```python
from build123d import *

# Parameters (mm, degrees)
SZKIC2_R                   = 3.3
SZKIC2_R_2                 = 8
WYTNIJ_WYCI_GNI_CIE1_DEPTH = 56.569775958


with BuildPart() as part:
    # Szkic1 → Obrót1 (revolve)
    with BuildSketch(Plane(origin=(0, 0, 0), x_dir=(0, 0, -1), z_dir=(1, 0, 0)), mode=Mode.PRIVATE) as obr_t1_sk:
        Polygon((0, 0), (44, 0), (44, 14), (10, 14), (10, 24), (0, 24), align=None)
    revolve(obr_t1_sk.sketch.rotate(Axis((0, 0, 0), (0, 0, -1)), 90), axis=Axis((0, 0, 0), (0, 0, -1)))

    # Szkic2 → Wytnij-wyciągnięcie1 (cut, through all)
    with BuildSketch(Plane.XY):
        with Locations((-13.435028843, 13.435028843)):
            Circle(SZKIC2_R)
        with Locations((0, 19)):
            Circle(SZKIC2_R)
        with Locations((13.435028843, 13.435028843)):
            Circle(SZKIC2_R)
        Circle(SZKIC2_R_2)
        with BuildLine():
            Line((-20, 13.266499161), (-20, -13.266499161))
            ThreePointArc((-20, -13.266499161), (-24, 0), (-20, 13.266499161))
        make_face()
        with BuildLine():
            Line((20, -13.266499161), (20, 13.266499161))
            ThreePointArc((20, 13.266499161), (24, 0), (20, -13.266499161))
        make_face()
    wytnij_wyci_gni_cie1 = extrude(amount=-WYTNIJ_WYCI_GNI_CIE1_DEPTH, mode=Mode.SUBTRACT)

    # Lustro1: Wytnij-wyciągnięcie1 across plane
    add(wytnij_wyci_gni_cie1.mirror(Plane.ZX), mode=Mode.SUBTRACT)


solid = part.part
```
The model under review builds one solid part; all positions refer to its coordinate system, in mm. A direction names the side the tool comes from. Coordinates: 2 decimals unless noted, no trailing zeros. Write each loop counter-clockwise with the first axis right and the second up, starting at its lowest first coordinate (ties: lowest second). Pieces come first, ordered by that corner, then holes. Notation, with made-up numbers: (-28.75, -4.5) - (22.25, -4.5) arc R18 ccw to (22.25, 5.5) - close; hole circle Ø7 at (-20.75, -16.75). An arc over 180 degrees is marked (long way). Answer in a Markdown table with one row per item. Add a question column.
Q1. Draft analysis for pull direction Y (two halves, no side actions). For faces 1 (the face through (9, 0, 0)), 2 (the face through (-0.72, 15.78, -4.93)), 3 (the face through (6.5, 12.4, -26.8)), state which applies: +Y half, -Y half, draft (parallel to the pull), parting line (faces both ways), or undercut.
Q2. Consider section C-C on z = -35.5. Give the boundary of the cut face in (x, y), then the cut area to 3 significant figures.
Q3. For faces 4 (the face through (0, 24, -5)), 5 (the face through (14, 5, -10)), list the 3-axis set-ups (+Z, -Z, +X, -X, +Y, -Y) from which the entire face can be reached by the end or side of a thin tool; tool diameter is ignored.
Q4. Consider section B-B on y = 0. Give the boundary of the cut face in (x, z).
Q5. Clearance check with flat-ended pins moving along their axes: pin 1 (3 mm diameter, centred on x = 5, z = -21.5, fed in from -Y); pin 2 (1.5 mm diameter, centred on x = -3, z = -24.5, fed in from -Y); pin 3 (5.5 mm diameter, centred on x = 13.44, y = 13.44, fed in from -Z); pin 4 (6 mm diameter, centred on x = 3, z = -27, fed in from -Y). State where each tip first meets the part, or that it passes through.
Q6. To check wall thickness, follow line 1 along Y through (x, z) = (0, -3); line 2 along Y through (x, z) = (12.5, -4); line 3 along X through (y, z) = (13, -6). State the ranges of each line that lie inside material, in increasing order. Write a range as from..to.
Q7. Consider section A-A on x = 0. Give the boundary of the cut face in (y, z).
Q8. Consider section D-D on x = 6.5. Give the boundary of the cut face in (y, z), then the cut area to 3 significant figures.
Answers below:
| question | item | result |
|---|---|---|
| 1 | face 1 | draft |
| 1 | face 2 | undercut |
| 1 | face 3 | parting line |
| 2 | outline | circle Ø28 at (0, 0); hole circle Ø16 at (0, 0) |
| 2 | area | 415 mm² |
| 3 | face 4 | +Z, -Z, +Y |
| 3 | face 5 | -Z |
| 4 | outline | (-20, -10) - (-14, -10) - (-14, -44) - (-8, -44) - (-8, 0) - (-20, 0) - close; (8, -44) - (14, -44) - (14, -10) - (20, -10) - (20, 0) - (8, 0) - close |
| 5 | pin 1 | y = -13.56 |
| 5 | pin 2 | y = -13.82 |
| 5 | pin 3 | through |
| 5 | pin 4 | y = -14 |
| 6 | line 1 | -24..-22.3, -15.7..-8, 8..15.7, 22.3..24 |
| 6 | line 2 | -20.49..-16.6, -10.27..10.27, 16.6..20.49 |
| 6 | line 3 | -20..-16.71, -10.16..10.16, 16.71..20 |
| 7 | outline | (-24, -10) - (-22.3, -10) - (-22.3, 0) - (-24, 0) - close; (-15.7, -10) - (-14, -10) - (-14, -44) - (-8, -44) - (-8, 0) - (-15.7, 0) - close; (8, -44) - (14, -44) - (14, -10) - (15.7, -10) - (15.7, 0) - (8, 0) - close; (22.3, -10) - (24, -10) - (24, 0) - (22.3, 0) - close |
| 8 | outline | (-23.1, -10) - (-12.4, -10) - (-12.4, -44) - (-4.66, -44) - (-4.66, 0) - (-23.1, 0) - close; (4.66, -44) - (12.4, -44) - (12.4, -10) - (23.1, -10) - (23.1, 0) - (4.66, 0) - close |
| 8 | area | 895 mm² |
